```python
from build123d import *

# Parameters (mm, degrees)
F0_W     = 139.7
F0_H     = 66.04
F1_DEPTH = 40.64
F2_W     = 99.06
F2_H     = 38.1
F3_DEPTH = 31.242
F4_R     = 5.08


with BuildPart() as f1:
    # F0 (on Top) → F1 (new body)
    with BuildSketch(Plane.XY):
        with Locations((-57.2554800045, -25.2220156343)):
            Rectangle(F0_W, F0_H)
    extrude(amount=F1_DEPTH)

    # F2 (on face) → F3 (join)
    with BuildSketch(Plane.XY.offset(40.64)):
        Polygon((-106.7854800045, 7.7979843657), (-127.1054800045, 7.7979843657), (-127.1054800045, -58.2420156343), (-106.7854800045, -58.2420156343), (-106.7854800045, -30.3020156343), align=None)
        Polygon((12.5945199955, 7.7979843657), (-7.7254800045, 7.7979843657), (-7.7254800045, -30.3020156343), (-7.7254800045, -58.2420156343), (12.5945199955, -58.2420156343), align=None)
        with Locations((-57.2554800045, -11.2520156343)):
            Rectangle(F2_W, F2_H)
    extrude(amount=F3_DEPTH)

    # F4
    f4_edges = [f1.edges().sort_by_distance(p)[0] for p in [
        (-57.25548, -30.302016, 71.882),
        (-7.72548, -44.272016, 71.882),
        (-106.78548, -44.272016, 71.882),
        (2.43452, -58.242016, 71.882),
        (12.59452, -25.222016, 71.882),
        (-116.94548, -58.242016, 71.882),
        (-127.10548, -25.222016, 71.882),
        (-57.25548, 7.797984, 71.882),
        (12.59452, -58.242016, 35.941),
        (-7.72548, -58.242016, 56.261),
        (-57.25548, -58.242016, 40.64),
        (-57.25548, -30.302016, 40.64),
        (-106.78548, -58.242016, 56.261),
        (-127.10548, -58.242016, 35.941),
        (-57.25548, -58.242016, 0),
        (-127.10548, -25.222016, 0),
        (-57.25548, 7.797984, 0),
        (-127.10548, 7.797984, 35.941),
        (12.59452, 7.797984, 35.941),
        (12.59452, -25.222016, 0),
    ]]
    fillet(f4_edges, radius=F4_R)


solid = f1.part
```
Source: CAD feature listing. Evaluate the final solid. Frame: model axes, mm. A direction names the side the tool comes from. Round coordinates to 2 decimals unless told otherwise and drop trailing zeros. Write each loop counter-clockwise with the first axis right and the second up, starting at its lowest first coordinate (ties: lowest second). Pieces come first, ordered by that corner, then holes. Notation, with made-up numbers: M -1,64.5 L 26,64.5 A25 ccw 26,87.5 Z; hole C -20,48 d3. An arc over 180 degrees is marked long. Use CSV: the item, a comma, the result in double quotes. Start each with the question number.
Q1. Cut plane A-A on y = -43. Output: boundary loops of the cut face in (x, z).
Q2. Access query for faces 5 (the face through (-58, -25, 0)), 6 (the face through (-108.31, -56.79, 51.4)). Directions: +Z, -Z, +X, -X, +Y, -Y. A direction counts if a zero-diameter tool reaches every point of the face in a straight line with its end or side. Return the directions, or none.
Q3. Pull-direction query (X, two-part tool) for faces 1 (the face through (-106.785, -42, 54)), 2 (the face through (-125.66, -24.83, 1.53)), 3 (the face through (-58, -30.302, 56)), 4 (the face through (-58, -19, 71.882)); classes: +X half, -X half, draft (parallel to the pull), parting line (faces both ways), or undercut.
Q4. First-contact query: P1, Ø9, axis at x = -73, y = -47, coming from the +Z side; P2, Ø3, axis at x = -65, z = 52, coming from the -Y side; P3, Ø1.5, axis at x = -9, z = 45, coming from the -Y side. Flat tips, straight axial feed; report the tip coordinate or a pass-through.
Q5. Cut plane B-B on x = -22. Output: boundary loops of the cut face in (y, z), plus the area to 3 significant figures.
Q6. Line query: line 1 (Z direction, x = -22, y = -51); line 2 (Y direction, x = -102, z = 61); line 3 (Y direction, x = -25.5, z = 3). Output: solid intervals per line, ascending. Write a range as from..to.
Q7. Cut plane C-C on z = 62. Output: boundary loops of the cut face in (x, y).
Results found:
1,outline,"M -127.11,5.08 A5.08 ccw -122.03,0 L 7.51,0 A5.08 ccw 12.59,5.08 L 12.59,66.8 A5.08 ccw 7.51,71.88 L -2.65,71.88 A5.08 ccw -7.73,66.8 L -7.73,40.64 L -106.79,40.64 L -106.79,66.8 A5.08 ccw -111.87,71.88 L -122.03,71.88 A5.08 ccw -127.11,66.8 Z"
2,face 5,"-Z, +X, -X, +Y, -Y"
2,face 6,"+Z, -Y"
3,face 1,"undercut"
3,face 2,"-X half"
3,face 3,"undercut"
3,face 4,"draft"
4,P1,"z = 40.64"
4,P2,"y = -30.3"
4,P3,"y = -30.52"
5,outline,"M -58.24,5.08 A5.08 ccw -53.16,0 L 2.72,0 A5.08 ccw 7.8,5.08 L 7.8,66.8 A5.08 ccw 2.72,71.88 L -25.22,71.88 A5.08 ccw -30.3,66.8 L -30.3,45.72 A5.08 cw -35.38,40.64 L -53.16,40.64 A5.08 ccw -58.24,35.56 Z"
5,area,"3,850 mm^2"
6,line 1,"0..40.64"
6,line 2,"-30.3..7.8"
6,line 3,"-57.8..7.35"
7,outline,"M -127.11,-53.16 A5.08 ccw -122.03,-58.24 L -111.87,-58.24 A5.08 ccw -106.79,-53.16 L -106.79,-30.3 L -7.73,-30.3 L -7.73,-53.16 A5.08 ccw -2.65,-58.24 L 7.51,-58.24 A5.08 ccw 12.59,-53.16 L 12.59,2.72 A5.08 ccw 7.51,7.8 L -122.03,7.8 A5.08 ccw -127.11,2.72 Z"
